```python
from build123d import *

# Parameters (mm, degrees)
SKETCH2_W                          = 42.672
SKETCH2_H                          = 35.56
SKETCH2_R                          = 12.7
BOSS_EXTRUDE1_DEPTH                = 12.7
TAP_DRILL_FOR_6_32_TAP1_AT_2_COUNT = 2
TAP_DRILL_FOR_6_32_TAP1_AT_2_PITCH = 27.94
TAP_DRILL_FOR_6_32_TAP1_AT_3_COUNT = 2
TAP_DRILL_FOR_6_32_TAP1_AT_3_PITCH = 6.604
TAP_DRILL_FOR_6_32_TAP1_AT_4_COUNT = 2
TAP_DRILL_FOR_6_32_TAP1_AT_4_PITCH = 28.709866179


with BuildPart() as part:
    # Sketch2 → Boss-Extrude1 (new body)
    with BuildSketch(Plane.XY):
        Rectangle(SKETCH2_W, SKETCH2_H)
        Circle(SKETCH2_R, mode=Mode.SUBTRACT)
    extrude(amount=BOSS_EXTRUDE1_DEPTH)

    # Sketch4 → Tap Drill for #6-32 Tap1 (revolve, cut)
    with BuildSketch(Plane(origin=(21.336, 13.97, 3.048), x_dir=(0, 0, -1), z_dir=(0, 1, 0))):
        Polygon((0, 0), (0, 7.16269403), (1.35255, 6.35), (1.35255, 0), align=None)
    tap_drill_for_6_32_tap1 = revolve(axis=Axis((27.686, 13.97, 3.048), (-1, 0, 0)), mode=Mode.SUBTRACT)

    # Tap Drill for #6-32 Tap1 at 2: Tap Drill for #6-32 Tap1 ×2
    with Locations(*[(0, -i * TAP_DRILL_FOR_6_32_TAP1_AT_2_PITCH, 0) for i in range(1, TAP_DRILL_FOR_6_32_TAP1_AT_2_COUNT)]):
        add(tap_drill_for_6_32_tap1, mode=Mode.SUBTRACT)

    # Tap Drill for #6-32 Tap1 at 3: Tap Drill for #6-32 Tap1 ×2
    with Locations(*[(0, 0, i * TAP_DRILL_FOR_6_32_TAP1_AT_3_PITCH) for i in range(1, TAP_DRILL_FOR_6_32_TAP1_AT_3_COUNT)]):
        add(tap_drill_for_6_32_tap1, mode=Mode.SUBTRACT)

    # Tap Drill for #6-32 Tap1 at 4: Tap Drill for #6-32 Tap1 ×2
    with Locations(*[Vector(0, -0.9731846127764102, 0.23002545392896967) * (i * TAP_DRILL_FOR_6_32_TAP1_AT_4_PITCH) for i in range(1, TAP_DRILL_FOR_6_32_TAP1_AT_4_COUNT)]):
        add(tap_drill_for_6_32_tap1, mode=Mode.SUBTRACT)

    # Mirror1: Tap Drill for #6-32 Tap1 across plane
    add(tap_drill_for_6_32_tap1.mirror(Plane(origin=(0, 0, 0), x_dir=(0, 0, 1), z_dir=(1, 0, 0))), mode=Mode.SUBTRACT)

    # Mirror1 copy 1 sketch → Mirror1 copy 1 (revolve, cut)
    with BuildSketch(Plane(origin=(-21.336, -13.97, 3.048), x_dir=(0, 0, -1), z_dir=(0, 1, 0))):
        Polygon((0, 0), (0, -7.16269403), (1.35255, -6.35), (1.35255, 0), align=None)
    revolve(axis=Axis((-27.686, -13.97, 3.048), (-1, 0, 0)), mode=Mode.SUBTRACT)

    # Mirror1 copy 2 sketch → Mirror1 copy 2 (revolve, cut)
    with BuildSketch(Plane(origin=(-21.336, 13.97, 9.652), x_dir=(0, 0, -1), z_dir=(0, 1, 0))):
        Polygon((0, 0), (0, -7.16269403), (1.35255, -6.35), (1.35255, 0), align=None)
    revolve(axis=Axis((-27.686, 13.97, 9.652), (-1, 0, 0)), mode=Mode.SUBTRACT)

    # Mirror1 copy 3 sketch → Mirror1 copy 3 (revolve, cut)
    with BuildSketch(Plane(origin=(-21.336, -13.97, 9.652), x_dir=(0, 0, -1), z_dir=(0, 1, 0))):
        Polygon((0, 0), (0, -7.16269403), (1.35255, -6.35), (1.35255, 0), align=None)
    revolve(axis=Axis((-27.686, -13.97, 9.652), (-1, 0, 0)), mode=Mode.SUBTRACT)


solid = part.part
```
Here's how the part is built. I have some questions about the finished solid (model axes, mm). A direction names the side the tool comes from. Round coordinates to 2 decimals unless told otherwise and drop trailing zeros. Write each loop counter-clockwise with the first axis right and the second up, starting at its lowest first coordinate (ties: lowest second). Pieces come first, ordered by that corner, then holes. Notation, with made-up numbers: M -37,86.25 L 20,86.25 A26 ccw 20,103.25 Z; hole C 26.25,45 d5. An arc over 180 degrees is marked long. Answer as CSV lines item,"result". Start each with the question number.
1. Thinking about a two-plate mould opening in Y: for faces 4 (the flat face through (-5, 12, 0)), 5 (the conical face through (14.314, -13.741, 3.099)), 6 (the flat face through (0, -17.78, 6)), which applies, released by +Y, released by -Y, zero draft, split by the parting line, or undercut?
2. On a 3-axis mill with a long thin cutter (end or side, diameter ignored), from which of +Z, -Z, +X, -X, +Y, -Y can I reach the whole of each face in a straight line? I mean faces 1 (the cylindrical face through (-18.21, -14.88, 10.65)), 2 (the cylindrical face through (18.21, -15.31, 3.22)), 3 (the flat face through (-5, 12, 12.7)). Say none if no direction works.
3. I need wall thicknesses on probe 1 along Z at (x, y) = (19.25, -13.97); probe 2 along X at (y, z) = (-0.5, 10); probe 3 along Y at (x, z) = (0, 2.25). Which ranges of each line are inside material? Lowest first, please.
4. Suppose I cut it at A-A on x = -17.5. Write out the boundary of the cut face in (y, z).
5. I'm going to push flat-ended pins straight in: pin 1 Ø2 at (y, z) = (-13.97, 3.048) entering from -X; pin 2 Ø2.5 at (y, z) = (13.97, 9.652) entering from -X; pin 3 Ø2 at (y, z) = (-13.97, 9.652) entering from +X. Where does each tip first touch, or does it pass through?
6. Suppose I cut it at C-C on y = 2.5. Write out the boundary of the cut face in (x, z), then the cut area to 3 significant figures.
7. Suppose I cut it at B-B on z = 5.25. Write out the boundary of the cut face in (x, y), then the cut area to 3 significant figures.
8. Suppose I cut it at D-D on x = 4. Write out the boundary of the cut face in (y, z), then the cut area to 3 significant figures.
Check result:
1,face 4,"zero draft"
1,face 5,"undercut"
1,face 6,"released by -Y"
2,face 1,"-X"
2,face 2,"+X"
2,face 3,"+Z, +X, -X, +Y, -Y"
3,probe 1,"z = 0 to 1.7, 4.4 to 8.3, 11 to 12.7"
3,probe 2,"x = -21.34 to -12.69, 12.69 to 21.34"
3,probe 3,"y = -17.78 to -12.7, 12.7 to 17.78"
4,outline,"M -17.78,0 L 17.78,0 L 17.78,12.7 L -17.78,12.7 Z; hole C -13.97,3.05 d2.71; hole C -13.97,9.65 d2.71; hole C 13.97,3.05 d2.71; hole C 13.97,9.65 d2.71"
5,pin 1,"stops at x = -14.77"
5,pin 2,"stops at x = -14.92"
5,pin 3,"stops at x = 14.77"
6,outline,"M -21.34,0 L -12.45,0 L -12.45,12.7 L -21.34,12.7 Z; M 12.45,0 L 21.34,0 L 21.34,12.7 L 12.45,12.7 Z"
6,area,"226 mm2"
7,outline,"M -21.34,-17.78 L 21.34,-17.78 L 21.34,17.78 L -21.34,17.78 Z; hole C 0,0 d25.4"
7,area,"1,010 mm2"
8,outline,"M -17.78,0 L -12.05,0 L -12.05,12.7 L -17.78,12.7 Z; M 12.05,0 L 17.78,0 L 17.78,12.7 L 12.05,12.7 Z"
8,area,"145 mm2"
